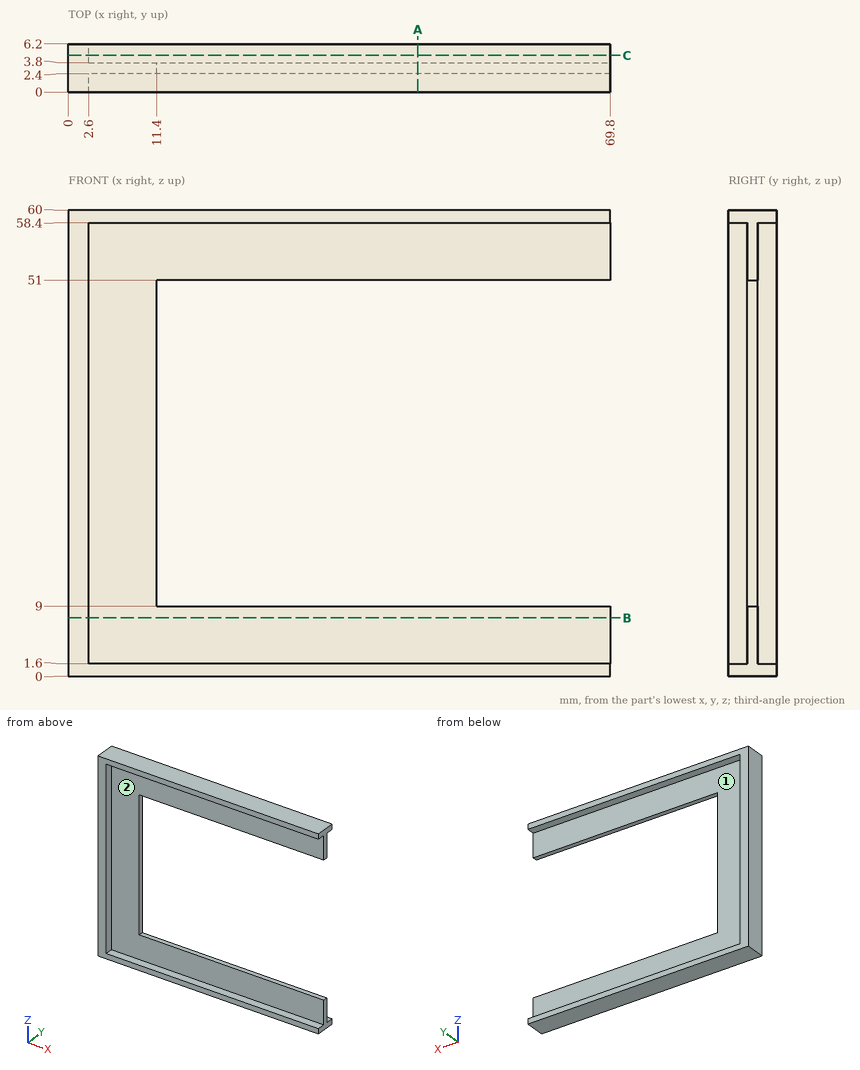
Source: three-view drawing plus pictorial views. Frame: mm from the lowest corner of the part. A direction names the side the tool comes from. Coordinates: 2 decimals unless noted, no trailing zeros. Order: outer loops, then holes, each group sorted by start corner. A loop starts at its lowest first (then second) coordinate and runs counter-clockwise, first axis right, second up. Notation, with made-up numbers: M 61.5,-16.5 L 120.5,-16.5 A17 ccw 120.5,-9.5 Z; hole C -11,-28 d3. An arc over 180 degrees is marked long. Answer in a Markdown table with one row per item.
(1) Contact query for flat-ended pins moving along their axis: pin 1 Ø0.7 at (x, y) = (51.5, 4.5) entering from -Z; pin 2 Ø3 at (y, z) = (4, 44) entering from +X; pin 3 Ø0.7 at (y, z) = (4.5, 27) entering from +X; pin 4 Ø5 at (x, z) = (11, 48.5) entering from -Y. Output: stop coordinate, or through.
Numbers:
| item | result |
|---|---|
| pin 1 | stops at z = 0 |
| pin 2 | stops at x = 11.4 |
| pin 3 | stops at x = 2.6 |
| pin 4 | stops at y = 2.4 |
(2) Material intervals for line 1 (Z direction, x = 13, y = 4.5); line 2 (Z direction, x = 40, y = 3); line 3 (X direction, y = 5.5, z = 36), sorted ascending. Write a range as [from, to].
Numbers:
| item | result |
|---|---|
| line 1 | z = [0, 1.6], [58.4, 60] |
| line 2 | z = [0, 9], [51, 60] |
| line 3 | x = [0, 2.6] |
(3) Section query C-C, the plane y = 4.75. Output: boundary loops of the cut face in (x, z).
Numbers:
| item | result |
|---|---|
| outline | M 0,0 L 69.8,0 L 69.8,1.6 L 2.6,1.6 L 2.6,58.4 L 69.8,58.4 L 69.8,60 L 0,60 Z |
(4) Access query for the marked faces 1 and 2. Directions: +Z, -Z, +X, -X, +Y, -Y. A direction counts if a zero-diameter tool reaches every point of the face in a straight line with its end or side. Return the directions, or none.
Numbers:
| item | result |
|---|---|
| face 1 | +X, +Y |
| face 2 | +X, -Y |
(5) Section query A-A, the plane x = 45. Output: boundary loops of the cut face in (y, z).
Numbers:
| item | result |
|---|---|
| outline | M 0,0 L 6.2,0 L 6.2,1.6 L 3.8,1.6 L 3.8,9 L 2.4,9 L 2.4,1.6 L 0,1.6 Z; M 0,58.4 L 2.4,58.4 L 2.4,51 L 3.8,51 L 3.8,58.4 L 6.2,58.4 L 6.2,60 L 0,60 Z |
(6) Section query B-B, the plane z = 7.5. Output: boundary loops of the cut face in (x, y), plus the area to 3 significant figures.
Numbers:
| item | result |
|---|---|
| outline | M 0,0 L 2.6,0 L 2.6,2.4 L 69.8,2.4 L 69.8,3.8 L 2.6,3.8 L 2.6,6.2 L 0,6.2 Z |
| area | 110 mm^2 |
